```python
from build123d import *

# Parameters (mm, degrees)
SKETCH_W        = 38
SKETCH_H        = 47.15
PAD_DEPTH       = 7
SKETCH001_R     = 1.5
POCKET_DEPTH    = 12
FILLET_R        = 4
SKETCH002_W     = 18
SKETCH002_H     = 34.5
POCKET001_DEPTH = 2
SKETCH003_W     = 10.28814
SKETCH003_H     = 13.233085
POCKET002_DEPTH = 2
SKETCH004_R     = 2
POCKET003_DEPTH = 4


with BuildPart() as part:
    # Sketch → Pad (new body)
    with BuildSketch(Plane.XY):
        Rectangle(SKETCH_W, SKETCH_H)
    extrude(amount=PAD_DEPTH)

    # Sketch001 (on Face4 of Pad) → Pocket (cut)
    with BuildSketch(Plane(origin=(0, 23.575, 0), x_dir=(-1, 0, 0), z_dir=(0, 1, 0))):
        with Locations((-12.075, 3.5)):
            Circle(SKETCH001_R)
        with Locations((12.075, 3.5)):
            Circle(SKETCH001_R)
    extrude(amount=-POCKET_DEPTH, mode=Mode.SUBTRACT)

    # Fillet
    fillet_edges = [part.edges().sort_by_distance(p)[0] for p in [
        (-19, 23.575, 3.5),
        (19, 23.575, 3.5),
    ]]
    fillet(fillet_edges, radius=FILLET_R)

    # Sketch002 (on Face5 of Fillet) → Pocket001 (cut)
    with BuildSketch(Plane.XY.offset(7)):
        with Locations((0, -6.325)):
            Rectangle(SKETCH002_W, SKETCH002_H)
    extrude(amount=-POCKET001_DEPTH, mode=Mode.SUBTRACT)

    # Sketch003 (on Face5 of Pocket001) → Pocket002 (cut)
    with BuildSketch(Plane.XY.offset(7)):
        with Locations((-0.070341, 16.958458)):
            Rectangle(SKETCH003_W, SKETCH003_H)
    extrude(amount=-POCKET002_DEPTH, mode=Mode.SUBTRACT)

    # Sketch004 (on Face20 of Pocket002) → Pocket003 (cut)
    with BuildSketch(Plane.XY.offset(5)):
        with Locations((-5.25, -0.575)):
            Circle(SKETCH004_R)
        with Locations((5.25, -0.575)):
            Circle(SKETCH004_R)
    extrude(amount=-POCKET003_DEPTH, mode=Mode.SUBTRACT)


solid = part.part
```
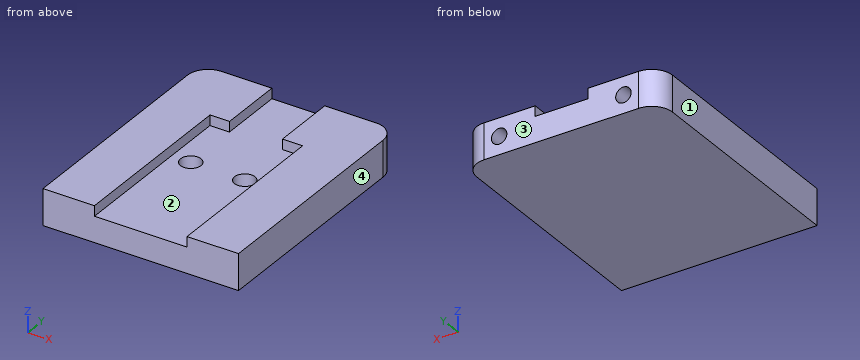
Check sheet for the modelled part. Datum: model origin and axes. Units: mm. Face numbers are marked on the shaded views. Give positions to 0.01 mm unless a question says otherwise; leave off trailing zeros. Write each loop counter-clockwise with the first axis right and the second up, starting at its lowest first coordinate (ties: lowest second). Pieces come first, ordered by that corner, then holes.
Item 1: Cross-section at C-C (z = 2.75). Enter the section's corners in (x, y) (3 decimals).
Item 2: Cross-section at B-B (y = -15.5). Enter the section's corners in (x, z), and give its area (3 significant figures).
Item 3: Cross-section at A-A (z = 6.25). Enter the section's corners in (x, y) (3 decimals).
Item 4: Cross-section at D-D (x = -4.5). Enter the section's corners in (y, z) (3 decimals).
Item 5: Gauge pin test, flat ends, axial feed: pin 1 (4 mm diameter, centred on x = 5, y = 5.5, fed in from +Z); pin 2 (2 mm diameter, centred on x = 4.5, y = 0, fed in from +Z); pin 3 (1.6 mm diameter, centred on x = -7.5, z = 6, fed in from -Y) (3 decimals). Record the tip position at first contact, or that the pin passes through.
Item 6: Draft check along X on the marked faces 1, 2, 3 and 4. Enter one of: released by +X, released by -X, zero draft, split by the parting line, or undercut.
Item 7: Scan lines: L1, parallel to X at y = 1, z = 6.75; L2, parallel to Y at x = 5.25, z = 4.05 (3 decimals); L3, parallel to Z at x = -12, y = 18.5. Record each from-to range of solid material in increasing order.
Report:
1. outline: (-19, -23.575) - (19, -23.575) - (19, 19.575) arc R4 ccw to (15, 23.575) - (13.374, 23.575) - (13.374, 11.575) - (10.776, 11.575) - (10.776, 23.575) - (-10.776, 23.575) - (-10.776, 11.575) - (-13.374, 11.575) - (-13.374, 23.575) - (-15, 23.575) arc R4 ccw to (-19, 19.575) - close; hole circle Ø4 at (-5.25, -0.575); hole circle Ø4 at (5.25, -0.575)
2. outline: (-19, 0) - (19, 0) - (19, 7) - (9, 7) - (9, 5) - (-9, 5) - (-9, 7) - (-19, 7) - close
2. area: 230 mm2
3. outline: (-19, -23.575) - (-9, -23.575) - (-9, 10.925) - (-5.214, 10.925) - (-5.214, 23.575) - (-15, 23.575) arc R4 ccw to (-19, 19.575) - close; (5.074, 10.925) - (9, 10.925) - (9, -23.575) - (19, -23.575) - (19, 19.575) arc R4 ccw to (15, 23.575) - (5.074, 23.575) - close
4. outline: (-23.575, 0) - (23.575, 0) - (23.575, 5) - (1.279, 5) - (1.279, 1) - (-2.429, 1) - (-2.429, 5) - (-23.575, 5) - close
5. pin 1: stops at z = 5
5. pin 2: stops at z = 1
5. pin 3: stops at y = 10.925
6. face 1: released by -X
6. face 2: undercut
6. face 3: zero draft
6. face 4: released by +X
7. L1: x = -19 to -9, 9 to 19
7. L2: y = -23.575 to -2.575, 1.425 to 23.575
7. L3: z = 0 to 2, 5 to 7
